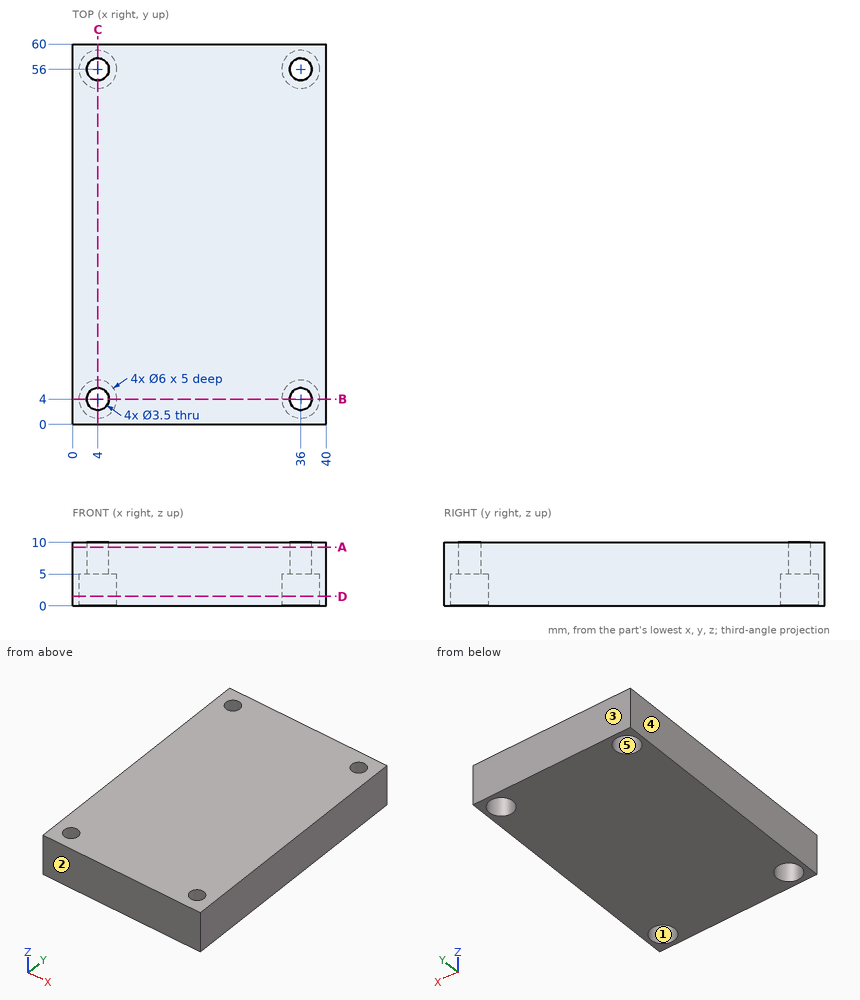
The drawing under review shows one solid part. Ordinate dimensions are in mm from its lowest x, y, z. A direction names the side the tool comes from. Coordinates: 2 decimals unless noted, no trailing zeros. Order: outer loops, then holes, each group sorted by start corner. A loop starts at its lowest first (then second) coordinate and runs counter-clockwise, first axis right, second up. Notation, with made-up numbers: (37, -1.75) -> (71, -1.75) arc R22 cw to (71, 8.25) -> close; hole circle Ø11 at (66, 44). An arc over 180 degrees is marked (long way). Use CSV: the item, a comma, the result in double quotes. Start each with the question number.
Item 1: We need section B-B, the plane y = 4. Give the boundary of the cut face in (x, z), then the cut area to 3 significant figures.
Item 2: We need section D-D, the plane z = 1.5. Give the boundary of the cut face in (x, y), then the cut area to 3 significant figures.
Item 3: For the marked faces 1 and 2, list the 3-axis set-ups (+Z, -Z, +X, -X, +Y, -Y) from which the entire face can be reached by the end or side of a thin tool; tool diameter is ignored.
Item 4: Wall thickness on probe 1 along Y at (x, z) = (36, 8.45); probe 2 along X at (y, z) = (4, 6.85); probe 3 along Y at (x, z) = (4, 3.45): over which ranges is each line inside the solid? List them lowest first.
Item 5: Insertion check: pin 1 (5.5 mm diameter, centred on x = 36, y = 56, fed in from -Z); pin 2 (2 mm diameter, centred on x = 4, y = 56, fed in from -Z). Each pin has a flat end and moves straight along its axis. Give the tip position at first contact, or say it passes through.
Item 6: We need section C-C, the plane x = 4. Give the boundary of the cut face in (y, z), then the cut area to 3 significant figures.
Item 7: Draft analysis for pull direction X (two halves, no side actions). For the marked faces 3, 4 and 5, state which applies: pulls with the +X half, pulls with the -X half, needs draft (parallel to the pull), parting line crosses it, or undercut.
Item 8: We need section A-A, the plane z = 9.25. Give the boundary of the cut face in (x, y).
Derived:
1,outline,"(0, 0) -> (1, 0) -> (1, 5) -> (2.25, 5) -> (2.25, 10) -> (0, 10) -> close; (5.75, 5) -> (7, 5) -> (7, 0) -> (33, 0) -> (33, 5) -> (34.25, 5) -> (34.25, 10) -> (5.75, 10) -> close; (37.75, 5) -> (39, 5) -> (39, 0) -> (40, 0) -> (40, 10) -> (37.75, 10) -> close"
1,area,"305 mm^2"
2,outline,"(0, 0) -> (40, 0) -> (40, 60) -> (0, 60) -> close; hole circle Ø6 at (4, 4); hole circle Ø6 at (4, 56); hole circle Ø6 at (36, 4); hole circle Ø6 at (36, 56)"
2,area,"2,290 mm^2"
3,face 1,"-Z"
3,face 2,"+Z, -Z, +X, -X, -Y"
4,probe 1,"y = 0 to 2.25, 5.75 to 54.25, 57.75 to 60"
4,probe 2,"x = 0 to 2.25, 5.75 to 34.25, 37.75 to 40"
4,probe 3,"y = 0 to 1, 7 to 53, 59 to 60"
5,pin 1,"stops at z = 5"
5,pin 2,"passes through"
6,outline,"(0, 0) -> (1, 0) -> (1, 5) -> (2.25, 5) -> (2.25, 10) -> (0, 10) -> close; (5.75, 5) -> (7, 5) -> (7, 0) -> (53, 0) -> (53, 5) -> (54.25, 5) -> (54.25, 10) -> (5.75, 10) -> close; (57.75, 5) -> (59, 5) -> (59, 0) -> (60, 0) -> (60, 10) -> (57.75, 10) -> close"
6,area,"505 mm^2"
7,face 3,"needs draft"
7,face 4,"pulls with the -X half"
7,face 5,"undercut"
8,outline,"(0, 0) -> (40, 0) -> (40, 60) -> (0, 60) -> close; hole circle Ø3.5 at (4, 4); hole circle Ø3.5 at (4, 56); hole circle Ø3.5 at (36, 4); hole circle Ø3.5 at (36, 56)"
